Autodesk Inventor part; units mm, degrees
ref_plane "YZ Plane" through (0, 0, 0) normal (1, 0, 0) x (0, 1, 0)
ref_plane "XZ Plane" through (0, 0, 0) normal (0, 1, 0) x (-1, 0, 0)
ref_plane "XY Plane" through (0, 0, 0) normal (0, 0, 1) x (1, 0, 0)
sketch "Sketch1" plane through (0, 0, 0) normal (0, 1, 0) x (-1, 0, 0)
  line L0 (24, 51) -> (-24, 51)
  line L1 (-24, 51) -> (-24, -51)
  line L2 (-24, -51) -> (24, -51)
  line L3 (24, -51) -> (24, 51)
  line L4 (24, 51) -> (-24, -51) construction
  line L5 (-24, 51) -> (24, -51) construction
  point P0 (0, 0)
  dimension "d0" = 48
  dimension "d1" = 102
extrude "Extrusion1" add sketch "Sketch1" along normal blind 0.7
fillet "Fillet1" radius 7 4 edges at (-24, 0.35, 51) (24, 0.35, 51) (24, 0.35, -51) (-24, 0.35, -51)
sketch "Sketch2" plane through (0, 0.7, 0) normal (0, 1, 0) x (1, 0, 0)
  circle A0 centre (-17, 44) radius 2.1
  arc A1 (-17, 51) -> (-24, 44) centre (-17, 44) ccw construction
  circle A2 centre (17, 44) radius 2.1
  arc A3 (24, 44) -> (17, 51) centre (17, 44) ccw construction
  circle A4 centre (-17, -44) radius 2.1
  arc A5 (-24, -44) -> (-17, -51) centre (-17, -44) ccw construction
  circle A6 centre (17, -44) radius 2.1
  arc A7 (17, -51) -> (24, -44) centre (17, -44) ccw construction
  point P0 (0, 0)
  dimension "d5" = 4.2
  dimension "d6" = 4.2
  dimension "d7" = 4.2
  dimension "d8" = 4.2
extrude "Extrusion2" cut sketch "Sketch2" against normal through all
sketch "Sketch3" plane through (0, 0.7, 0) normal (0, 1, 0) x (1, 0, 0)
  line L0 (-19, -40) -> (19, -40)
  line L1 (19, -40) -> (19, 40)
  line L2 (19, 40) -> (-19, 40)
  line L3 (-19, 40) -> (-19, -40)
  line L4 (-19, -40) -> (19, 40) construction
  line L5 (19, -40) -> (-19, 40) construction
  point P0 (0, 0)
  dimension "d11" = 38
  dimension "d12" = 80
extrude "Extrusion3" cut sketch "Sketch3" against normal through all
fillet "Fillet2" radius 4 4 edges at (-19, 0.35, -40) (19, 0.35, -40) (19, 0.35, 40) (-19, 0.35, 40)
properties part number "GearBoxSpacers"
Verification items for the finished model (mm, model axes). A direction names the side the tool comes from. Coordinates: 2 decimals unless noted, no trailing zeros. Write each loop counter-clockwise with the first axis right and the second up, starting at its lowest first coordinate (ties: lowest second). Pieces come first, ordered by that corner, then holes. Notation, with made-up numbers: M -16,-32.75 L 5,-32.75 A5 ccw 5,-27.75 Z; hole C -22,81 d11. An arc over 180 degrees is marked long. Answer as a JSON object with one key per item and string values. Group by question number.
(1) Gauge pin test, flat end, axial feed: pin 1 (6.5 mm diameter, centred on x = 17, z = 44, fed in from +Y). Record the tip position at first contact, or that the pin passes through.
(2) Cross-section at A-A, the plane z = -19.5. Record the cut outline in (x, y).
(3) Cross-section at B-B, the plane x = 11.5. Record the cut outline in (y, z).
(4) Release check for a two-part mould opening along Z. For faces 1 (the face through (-22, 0.4, 48.9)), 2 (the face through (-17.859, 0.345, -38.797)), 3 (the face through (-21.9, 0.4, -49)) record: +Z half, -Z half, draft (parallel to the pull), parting line (faces both ways), or undercut.
(5) Material ranges on line 1 (X direction, y = 0.5, z = -44); line 2 (Z direction, x = -8, y = 0.2); line 3 (Z direction, x = -17, y = 0.3), recorded low to high.
(6) Tool access check on faces 4 (the face through (22, 0, 1)), 5 (the face through (-17.797, 0.345, 38.859)). Record the directions out of +Z, -Z, +X, -X, +Y, -Y that give a thin tool (end or side, any length) a straight path to the whole face; none if there is none.
Reply:
{
 "1": {"pin 1": "y = 0.7"},
 "2": {"outline": "M -24,0 L -19,0 L -19,0.7 L -24,0.7 Z; M 19,0 L 24,0 L 24,0.7 L 19,0.7 Z"},
 "3": {"outline": "M 0,-51 L 0.7,-51 L 0.7,-40 L 0,-40 Z; M 0,40 L 0.7,40 L 0.7,51 L 0,51 Z"},
 "4": {"face 1": "+Z half", "face 2": "undercut", "face 3": "-Z half"},
 "5": {"line 1": "-24 to -19.1, -14.9 to 14.9, 19.1 to 24", "line 2": "-51 to -40, 40 to 51", "line 3": "-51 to -46.1, -41.9 to -39.46, 39.46 to 41.9, 46.1 to 51"},
 "6": {"face 4": "+Z, -Z, +X, -X, -Y", "face 5": "+Y, -Y"}
}
